Model file for the job. Use its own axes, mm. Coordinates: 2 decimals unless noted, no trailing zeros. Loops run counter-clockwise (first coordinate to the right, second up) from the corner with the lowest first, then second, coordinate; pieces in that order, holes last.
from build123d import *

# Parameters (mm, degrees)
SKETCH1_W           = 86
SKETCH1_H           = 41
BOSS_EXTRUDE1_DEPTH = 1.3
SKETCH2_W           = 1.4
SKETCH2_H           = 20
SKETCH2_W_2         = 30
SKETCH2_H_2         = 1.4
BOSS_EXTRUDE2_DEPTH = 1.3
SKETCH3_W           = 1
SKETCH3_H           = 10
CUT_EXTRUDE1_DEPTH  = 50.524337451


with BuildPart() as part:
    # Sketch1 → Boss-Extrude1 (new body)
    with BuildSketch(Plane.XY):
        Rectangle(SKETCH1_W, SKETCH1_H)
        Polygon((-38, 18), (38, 18), (29.867102397, 0), (-32.132897603, 0), align=None, mode=Mode.SUBTRACT)
    extrude(amount=BOSS_EXTRUDE1_DEPTH)

    # Sketch2 → Boss-Extrude2 (add)
    with BuildSketch(Plane.XY.offset(1.3)):
        with Locations((-43.7, -0.75)):
            Rectangle(SKETCH2_W, SKETCH2_H)
        with Locations((43.7, -0.75)):
            Rectangle(SKETCH2_W, SKETCH2_H)
        with Locations((0, 21.2)):
            Rectangle(SKETCH2_W_2, SKETCH2_H_2)
        with Locations((0, -21.2)):
            Rectangle(SKETCH2_W_2, SKETCH2_H_2)
    extrude(amount=-BOSS_EXTRUDE2_DEPTH)

    # Sketch3 → Cut-Extrude1 (cut, through all)
    with BuildSketch(Plane.XY.offset(1.3)):
        with Locations((-10.5, -10.5)):
            Rectangle(SKETCH3_W, SKETCH3_H)
        with Locations((10.5, -10.5)):
            Rectangle(SKETCH3_W, SKETCH3_H)
    extrude(amount=-CUT_EXTRUDE1_DEPTH, mode=Mode.SUBTRACT)


solid = part.part
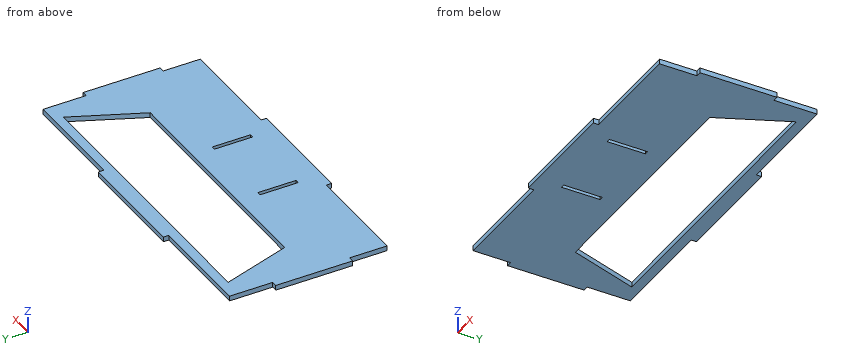
Q1. Drill centre lines: line 1 (X direction, y = -13.5, z = 1.1); line 2 (Y direction, x = -1.5, z = 0.3); line 3 (Y direction, x = -20, z = 0.75). Where is each one in solid material? Low to high.
Answers:
line 1: x = -43 to -11, -10 to 10, 11 to 43
line 2: y = -21.9 to 0, 18 to 21.9
line 3: y = -20.5 to 0, 18 to 20.5
Q2. Slice it at A-A (x = 29). List the corners of the cut face in (y, z), and give its area (3 significant figures).
Answers:
outline: (-20.5, 0) - (0, 0) - (0, 1.3) - (-20.5, 1.3) - close; (18, 0) - (20.5, 0) - (20.5, 1.3) - (18, 1.3) - close
area: 29.9 mm2
Q3. Slice it at B-B (y = -7). List the corners of the cut face in (x, z), and give its area (3 significant figures).
Answers:
outline: (-44.4, 0) - (-11, 0) - (-11, 1.3) - (-44.4, 1.3) - close; (-10, 0) - (10, 0) - (10, 1.3) - (-10, 1.3) - close; (11, 0) - (44.4, 0) - (44.4, 1.3) - (11, 1.3) - close
area: 113 mm2
Q4. Flat gauge pins, fed straight in: P1, Ø0.6, axis at x = 28.5, z = 0.5, coming from the +Y side; P2, Ø0.6, axis at x = 26.5, z = 0.5, coming from the -Y side. Where does each tip first touch, or does it go through?
Answers:
P1: stops at y = 20.5
P2: stops at y = -20.5
Q5. Slice it at C-C (z = 0.75). Count the separate pieces of the cut face and the enclosed holes in it, and give its area (3 significant figures).
Answers:
separate pieces: 1
enclosed holes: 3
area: 2,400 mm2
Q6. Slice it at D-D (x = 2). List the corners of the cut face in (y, z), and give its area (3 significant figures).
Answers:
outline: (-21.9, 0) - (0, 0) - (0, 1.3) - (-21.9, 1.3) - close; (18, 0) - (21.9, 0) - (21.9, 1.3) - (18, 1.3) - close
area: 33.5 mm2
